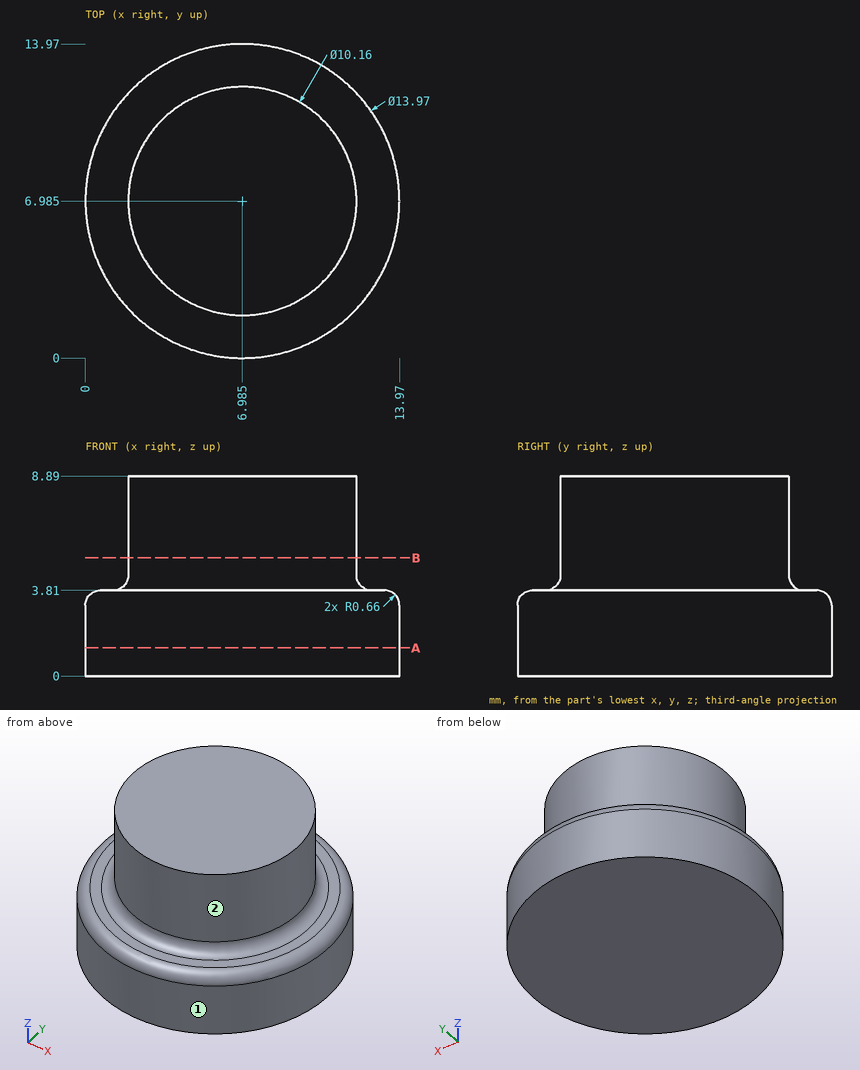
The figure shows three views and two pictorial views of one solid part (mm, origin at its lowest corner). Answer the questions. A direction names the side the tool comes from. Round coordinates to 2 decimals unless told otherwise and drop trailing zeros. Write each loop counter-clockwise with the first axis right and the second up, starting at its lowest first coordinate (ties: lowest second). Pieces come first, ordered by that corner, then holes. Notation, with made-up numbers: (14.25, 51.25) -> (48.25, 51.25) arc R21 cw to (48.25, 72.25) -> close; hole circle Ø6 at (66, 51). An arc over 180 degrees is marked (long way). Answer as a JSON object with one key per item and string values. Group by question number.
Q1. Straight lines are drawn through the part: line 1 along Z through (x, y) = (3.75, 1.5); line 2 along Y through (x, z) = (3.75, 8); line 3 along Y through (x, z) = (9, 6.75). For each, find the intervals that lie inside material, in ascending order.
Q2. Section A-A (z = 1.25) is taken. Write down the section's boundary in (x, y) (1 decimal).
Q3. Each of these flat-tipped pins is pushed along its axis until it touches: pin 1 Ø4 at (x, z) = (2, 2) entering from +Y; pin 2 Ø8 at (x, y) = (8.5, 1.5) entering from +Z; pin 3 Ø1 at (x, z) = (8.5, 1.5) entering from -Y. Where does it stop, or does it pass through?
Q4. Section B-B (z = 5.25) is taken. Write down the section's boundary in (x, y) (1 decimal).
Q5. Which of the six approach directions +Z, -Z, +X, -X, +Y, -Y give full straight-line access (tool end or side, diameter ignored) to the marked faces 1 and 2?
Check values:
{
 "1": {"line 1": "0 to 3.81", "line 2": "3.07 to 10.9", "line 3": "2.32 to 11.65"},
 "2": {"outline": "circle Ø14 at (7, 7)"},
 "3": {"pin 1": "y = 13.3", "pin 2": "z = 8.89", "pin 3": "y = 0.07"},
 "4": {"outline": "circle Ø10.2 at (7, 7)"},
 "5": {"face 1": "+Z, -Z", "face 2": "+Z"}
}
